from build123d import *

# Parameters (mm, degrees)
F2_SIZE = 2.286
F3_R    = 4.318


with BuildPart() as f1:
    # F0 (on Front) → F1 (revolve)
    with BuildSketch(Plane.XZ):
        Polygon((-17.131681, 0), (-22.225, 0), (-22.225, -28.448), (-18.161, -28.448), (-18.161, -24.675057), (-19.972013, -24.675057), (-19.972013, -22.796622), (-18.161, -22.796622), (-18.161, -2.265504), (-17.131681, -2.265504), align=None)
    revolve(axis=Axis((0, 0, -14.224), (0, 0, -1)))

    # F2
    f2_edges = [f1.edges().sort_by_distance(p)[0] for p in [
        (18.161, 0, -28.448),
    ]]
    chamfer(f2_edges, length=F2_SIZE)

    # F3
    f3_edges = [f1.edges().sort_by_distance(p)[0] for p in [
        (22.225, 0, 0),
    ]]
    fillet(f3_edges, radius=F3_R)


solid = f1.part
Model file for the job. Use its own axes, mm. A direction names the side the tool comes from. Coordinates: 2 decimals unless noted, no trailing zeros. Order: outer loops, then holes, each group sorted by start corner. A loop starts at its lowest first (then second) coordinate and runs counter-clockwise, first axis right, second up. Notation, with made-up numbers: (42, 58) -> (53, 58) arc R29 ccw to (53, 91) -> close; hole circle Ø5 at (74.25, 50). An arc over 180 degrees is marked (long way). Return JSON: item names as keys, results as strings. Group by question number.
Item 1: Wall check: line 1 along Y through (x, z) = (0, -15.25) (3 decimals); line 2 along X through (y, z) = (15.5, -7.5); line 3 along X through (y, z) = (1.5, -12.25). Give the ranges that are in metal, low to high. Write a range as [from, to].
Item 2: Tool access for faces 5 (the cylindrical face through (-9.763, 15.313, -25.408)), 6 (the cylindrical face through (-16.34, 5.15, -1.12)), 7 (the flat face through (4, -18, -24.675)): list every direction of +Z, -Z, +X, -X, +Y, -Y with a clear straight run to the whole face (end or side of a thin tool).
Item 3: Pull direction Z, two halves, no side cores. Call faces 1 (the flat face through (-7, -16, -2.266)), 2 (the cylindrical face through (-9.763, 15.313, -12.387)), 3 (the cylindrical face through (15.85, -12.15, -23.72)), 4 (the flat face through (15, -9, 0)): pulls with the +Z half, pulls with the -Z half, needs draft (parallel to the pull), parting line crosses it, or undercut.
Item 4: Saw through at C-C on z = -13.75. Write the cut outline in (x, y) (3 decimals).
Item 5: Saw through at A-A on y = 0. Write the cut outline in (x, z) (1 decimal).
Item 6: Flat gauge pins, fed straight in: P1, Ø12, axis at y = 7.5, z = -5.5, coming from the -X side; P2, Ø10, axis at x = -9, z = -20.5, coming from the -Y side; P3, Ø5, axis at x = -10.5, z = -20.5, coming from the -Y side; P4, Ø12, axis at x = -9, y = -8.5, coming from the +Z side. Where does each tip first touch, or does it go through?
Values found:
{
 "1": {"line 1": "y = [-22.225, -18.161], [18.161, 22.225]", "line 2": "x = [-15.93, -9.46], [9.46, 15.93]", "line 3": "x = [-22.17, -18.1], [18.1, 22.17]"},
 "2": {"face 5": "-Z", "face 6": "+Z, -Z", "face 7": "none"},
 "3": {"face 1": "pulls with the -Z half", "face 2": "needs draft", "face 3": "undercut", "face 4": "pulls with the +Z half"},
 "4": {"outline": "circle Ø44.45 at (0, 0); hole circle Ø36.322 at (0, 0)"},
 "5": {"outline": "(-22.2, -28.4) -> (-20.4, -28.4) -> (-18.2, -26.2) -> (-18.2, -24.7) -> (-20, -24.7) -> (-20, -22.8) -> (-18.2, -22.8) -> (-18.2, -2.3) -> (-17.1, -2.3) -> (-17.1, 0) -> (-17.9, 0) arc R4.3 ccw to (-22.2, -4.3) -> close; (17.1, -2.3) -> (18.2, -2.3) -> (18.2, -22.8) -> (20, -22.8) -> (20, -24.7) -> (18.2, -24.7) -> (18.2, -26.2) -> (20.4, -28.4) -> (22.2, -28.4) -> (22.2, -4.3) arc R4.3 ccw to (17.9, 0) -> (17.1, 0) -> close"},
 "6": {"P1": "stops at x = -22.17", "P2": "stops at y = -21.86", "P3": "stops at y = -20.74", "P4": "stops at z = 0"}
}
